Input: part model. Units: mm. Frame: model coordinates. Face numbers are marked on the shaded views. A direction names the side the tool comes from. Round coordinates to 2 decimals unless told otherwise and drop trailing zeros. Write each loop counter-clockwise with the first axis right and the second up, starting at its lowest first coordinate (ties: lowest second). Pieces come first, ordered by that corner, then holes. Notation, with made-up numbers: M -21.75,11 L 13.25,11 A37 cw 13.25,47 Z; hole C -17,85 d6. An arc over 180 degrees is marked long. Answer as CSV lines item,"result". Start each with the question number.
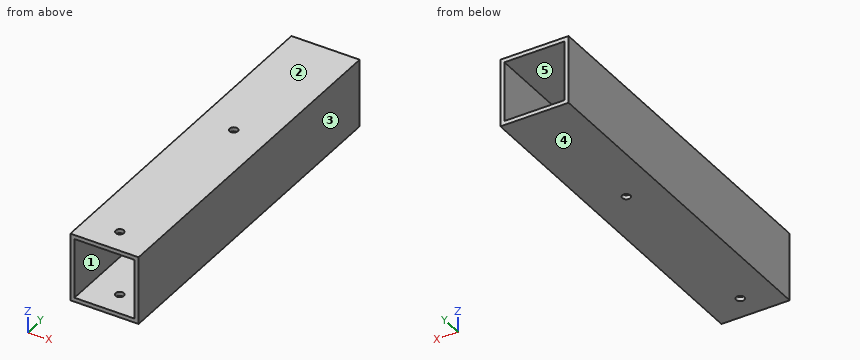
```python
from build123d import *

# Parameters (mm, degrees)
BOSS_EXTRUDE1_DEPTH      = 65
BOSS_EXTRUDE1_DEPTH_BACK = 65
SKETCH3_W                = 25
SKETCH3_H                = 25
SKETCH3_W_2              = 22
SKETCH3_H_2              = 22
SKETCH5_R                = 1.5
CUT_EXTRUDE2_DEPTH       = 25


with BuildPart() as part:
    # Sketch3 → Boss-Extrude1 (new, two sides: drawn at the far end of the back side and taken through both)
    with BuildSketch(Plane(origin=(0, 0, 0), x_dir=(1, 0, 0), z_dir=(0, 1, 0)).offset(-BOSS_EXTRUDE1_DEPTH_BACK)):
        Rectangle(SKETCH3_W, SKETCH3_H)
        Rectangle(SKETCH3_W_2, SKETCH3_H_2, mode=Mode.SUBTRACT)
    extrude(amount=BOSS_EXTRUDE1_DEPTH + BOSS_EXTRUDE1_DEPTH_BACK)

    # Sketch5 → Cut-Extrude2 (cut)
    with BuildSketch(Plane(origin=(0, 0, -12.5), x_dir=(-1, 0, 0), z_dir=(0, 0, -1))):
        with Locations((0, -56)):
            Circle(SKETCH5_R)
        with Locations((0, 11)):
            Circle(SKETCH5_R)
    extrude(amount=-CUT_EXTRUDE2_DEPTH, mode=Mode.SUBTRACT)


solid = part.part
```
Item 1: Cut plane C-C, the plane y = 11. Return loops of the section in (x, z), plus the area to 3 significant figures.
Item 2: Draft query along X for the marked faces 3, 4 and 5. Return one class per face: +X half, -X half, draft (parallel to the pull), parting line (faces both ways), or undercut.
Item 3: Cut plane B-B, the plane z = 9.25. Return loops of the section in (x, y).
Item 4: Cut plane D-D, the plane y = -21. Return loops of the section in (x, z), plus the area to 3 significant figures.
Item 5: Line query: line 1 (Y direction, x = 0, z = -11.9); line 2 (Z direction, x = -0.75, y = 8). Output: solid intervals per line, ascending. Write a range as [from, to].
Item 6: Pin query (flat end, axial travel): pin 1 Ø4 at (x, y) = (0, 11) entering from +Z. Return the tip coordinate at first contact, or that it passes through.
Item 7: Access query for the marked faces 1 and 2. Directions: +Z, -Z, +X, -X, +Y, -Y. A direction counts if a zero-diameter tool reaches every point of the face in a straight line with its end or side. Return the directions, or none.
Item 8: Cut plane A-A, the plane x = -3.5. Return loops of the section in (y, z), plus the area to 3 significant figures.
Results list:
1,outline,"M -12.5,-12.5 L -1.5,-12.5 L -1.5,-11 L -11,-11 L -11,11 L -1.5,11 L -1.5,12.5 L -12.5,12.5 Z; M 1.5,-12.5 L 12.5,-12.5 L 12.5,12.5 L 1.5,12.5 L 1.5,11 L 11,11 L 11,-11 L 1.5,-11 Z"
1,area,"132 mm²"
2,face 3,"+X half"
2,face 4,"draft"
2,face 5,"undercut"
3,outline,"M -12.5,-65 L -11,-65 L -11,65 L -12.5,65 Z; M 11,-65 L 12.5,-65 L 12.5,65 L 11,65 Z"
4,outline,"M -12.5,-12.5 L 12.5,-12.5 L 12.5,12.5 L -12.5,12.5 Z; hole M -11,-11 L 11,-11 L 11,11 L -11,11 Z"
4,area,"141 mm²"
5,line 1,"[-65, -57.5], [-54.5, 9.5], [12.5, 65]"
5,line 2,"[-12.5, -11], [11, 12.5]"
6,pin 1,"z = 12.5"
7,face 1,"+Y, -Y"
7,face 2,"+Z, +X, -X, +Y, -Y"
8,outline,"M -65,-12.5 L 65,-12.5 L 65,-11 L -65,-11 Z; M -65,11 L 65,11 L 65,12.5 L -65,12.5 Z"
8,area,"390 mm²"
